Geometry check sheet. Reference: drawing and pictorial views, mm from the part's lowest x, y, z. Coordinates: 2 decimals unless noted, no trailing zeros. Loops run counter-clockwise (first coordinate to the right, second up) from the corner with the lowest first, then second, coordinate; pieces in that order, holes last. Notation, with made-up numbers: (80, -2.5) - (86, -2.5) arc R11 ccw to (86, 13.5) - close; hole circle Ø7 at (-2.5, 15.25). An arc over 180 degrees is marked (long way). One line per item, written item: value.
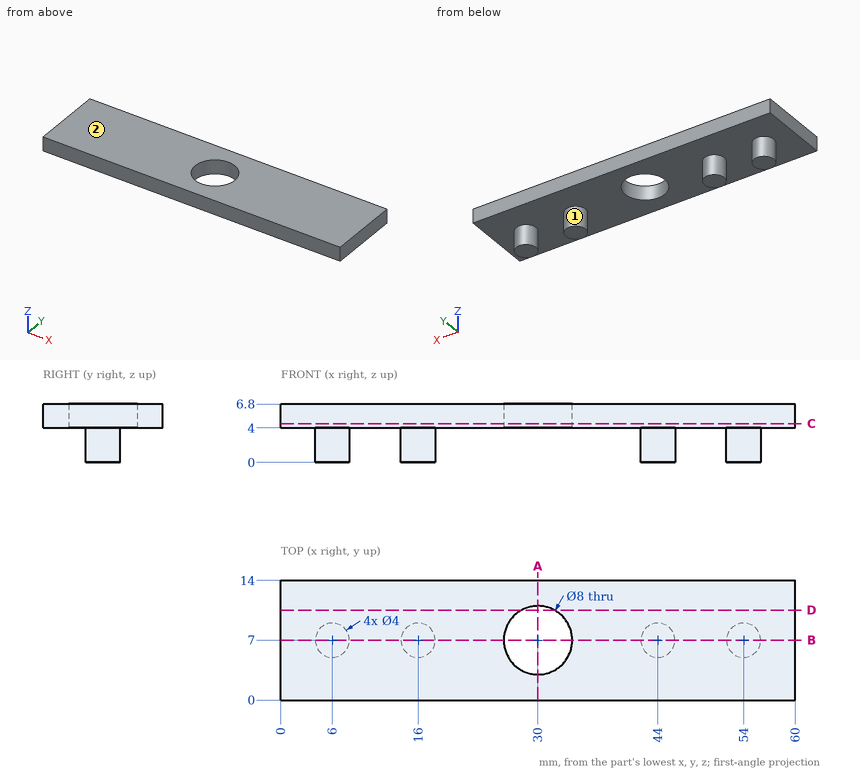
(1) Cross-section at B-B on y = 7. Record the cut outline in (x, z).
Reply:
outline: (0, 4) - (4, 4) - (4, 0) - (8, 0) - (8, 4) - (14, 4) - (14, 0) - (18, 0) - (18, 4) - (26, 4) - (26, 6.8) - (0, 6.8) - close; (34, 4) - (42, 4) - (42, 0) - (46, 0) - (46, 4) - (52, 4) - (52, 0) - (56, 0) - (56, 4) - (60, 4) - (60, 6.8) - (34, 6.8) - close
(2) Cross-section at C-C on z = 4.5. Record the cut outline in (x, y).
Reply:
outline: (0, 0) - (60, 0) - (60, 14) - (0, 14) - close; hole circle Ø8 at (30, 7)
(3) Material ranges on probe 1 along Y at (x, z) = (30, 5.25); probe 2 along Z at (x, y) = (39.5, 5.25); probe 3 along X at (y, z) = (6.5, 1.75), recorded low to high. Write a range as from..to.
Reply:
probe 1: 0..3, 11..14
probe 2: 4..6.8
probe 3: 4.06..7.94, 14.06..17.94, 42.06..45.94, 52.06..55.94
(4) Release check for a two-part mould opening along X. For the marked faces 1 and 2 record: pulls with the +X half, pulls with the -X half, needs draft (parallel to the pull), parting line crosses it, or undercut.
Reply:
face 1: undercut
face 2: needs draft
(5) Cross-section at D-D on y = 10.5. Record the cut outline in (x, z).
Reply:
outline: (0, 4) - (28.06, 4) - (28.06, 6.8) - (0, 6.8) - close; (31.94, 4) - (60, 4) - (60, 6.8) - (31.94, 6.8) - close
(6) Go/stop test with flat-tipped pins: pin 1 Ø7 at (x, y) = (30, 7) entering from +Z; pin 2 Ø7 at (x, y) = (37, 4.5) entering from -Z; pin 3 Ø1.5 at (y, z) = (6.5, 3) entering from -X. Record where each tip stops, or that it passes through.
Reply:
pin 1: through
pin 2: z = 4
pin 3: x = 4
(7) Cross-section at A-A on x = 30. Record the cut outline in (y, z), and give its area (3 significant figures).
Reply:
outline: (0, 4) - (3, 4) - (3, 6.8) - (0, 6.8) - close; (11, 4) - (14, 4) - (14, 6.8) - (11, 6.8) - close
area: 16.8 mm2
